Source: CAD feature listing. Evaluate the final solid. Frame: model axes, mm. Face numbers are marked on the shaded views. A direction names the side the tool comes from. Give positions to 0.01 mm unless a question says otherwise; leave off trailing zeros. Order: outer loops, then holes, each group sorted by start corner. A loop starts at its lowest first (then second) coordinate and runs counter-clockwise, first axis right, second up. Notation, with made-up numbers: M -22.5,33 L 34.5,33 A37 cw 34.5,69 Z; hole C 14.5,-28.5 d1. An arc over 180 degrees is marked long. Return JSON: item names as keys, results as strings.
from build123d import *
from build123d.topology import SkipClean

# Parameters (mm, degrees)
BOSS_EXTRUDE1_DEPTH = 19
SKETCH2_R           = 2.1
BOSS_EXTRUDE2_DEPTH = 1
SKETCH3_R           = 4.5
BOSS_EXTRUDE3_DEPTH = 1.5
SKETCH4_R           = 2.5
BOSS_EXTRUDE4_DEPTH = 2.5
BOSS_EXTRUDE5_DEPTH = 6


with BuildPart() as part:
    # Sketch1 → Boss-Extrude1 (new body)
    with BuildSketch(Plane(origin=(0, 0, 0), x_dir=(1, 0, 0), z_dir=(0, 1, 0))):
        with BuildLine():
            Line((-7.4, -17), (-7.4, -11.884443613))
            ThreePointArc((-7.4, -11.884443613), (0, 14), (7.4, -11.884443613))
            Line((7.4, -11.884443613), (7.4, -17))
            Line((7.4, -17), (-7.4, -17))
        make_face()
    extrude(amount=BOSS_EXTRUDE1_DEPTH)

    # Sketch2 → Boss-Extrude2 (add)
    # profile 1 of 2: a face of its own
    with BuildSketch(Plane.XZ):
        with BuildLine():
            Line((13.555441712, -3.5), (13.555441712, 3.5))
            Line((13.555441712, 3.5), (17.5, 3.5))
            ThreePointArc((17.5, 3.5), (21, 0), (17.5, -3.5))
            Line((17.5, -3.5), (13.555441712, -3.5))
        make_face()
        with Locations(Location((17.5, 0, 0), (0, 0, 90))):
            Circle(SKETCH2_R, mode=Mode.SUBTRACT)
    # profile 2 of 2: a face of its own
    with BuildSketch(Plane.XZ):
        with BuildLine():
            Line((-17.5, -3.5), (-13.555441712, -3.5))
            Line((-13.555441712, -3.5), (-13.555441712, 3.5))
            Line((-13.555441712, 3.5), (-17.5, 3.5))
            ThreePointArc((-17.5, 3.5), (-21, 0), (-17.5, -3.5))
        make_face()
        with Locations(Location((-17.5, 0, 0), (0, 0, 270))):
            Circle(SKETCH2_R, mode=Mode.SUBTRACT)
    extrude(amount=-BOSS_EXTRUDE2_DEPTH)

    # Sketch3 → Boss-Extrude3 (add)
    with BuildSketch(Plane.XZ):
        with Locations(Location((0, -8, 0), (0, 0, 90))):
            Circle(SKETCH3_R)
    extrude(amount=BOSS_EXTRUDE3_DEPTH)

    # Sketch4 → Boss-Extrude4 (add)
    with BuildSketch(Plane.XZ.offset(1.5)):
        with Locations(Location((0, -8, 0), (0, 0, 270))):
            Circle(SKETCH4_R)
    extrude(amount=BOSS_EXTRUDE4_DEPTH)

    # Sketch5 → Boss-Extrude5 (add)
    with SkipClean():  # the faces are left unmerged after this step: merging them gives an invalid solid
        with BuildSketch(Plane.XZ.offset(4)):
            with BuildLine():
                Line((-1.5, -10), (-1.5, -6))
                ThreePointArc((-1.5, -6), (0, -5.5), (1.5, -6))
                Line((1.5, -6), (1.5, -10))
                ThreePointArc((1.5, -10), (0, -10.5), (-1.5, -10))
            make_face()
        extrude(amount=BOSS_EXTRUDE5_DEPTH)


solid = part.part
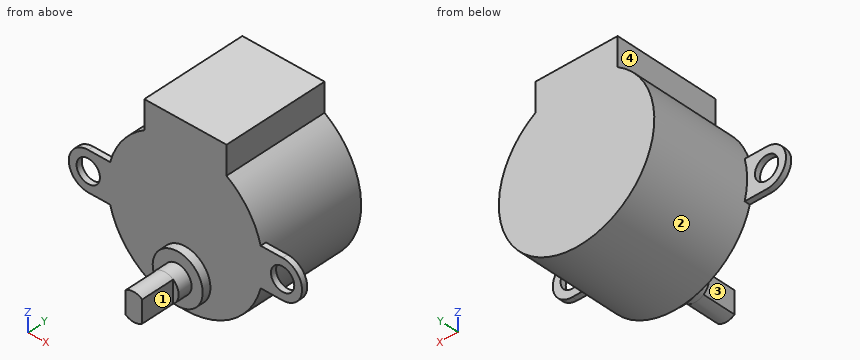
1. First-contact query: pin 1 (8 mm diameter, centred on y = 14.5, z = 4, fed in from -X); pin 2 (2 mm diameter, centred on y = -6, z = -8, fed in from +X); pin 3 (1.2 mm diameter, centred on y = -8.5, z = -8, fed in from -X). Flat tips, straight axial feed; report the tip coordinate or a pass-through.
Evaluation:
{"pin 1": "stops at x = -14", "pin 2": "stops at x = 1.5", "pin 3": "stops at x = -1.5"}
2. Section query C-C (x = -4). Return loops of the section in (y, z).
Evaluation:
{"outline": "M -1.5,-10.06 L 0,-10.06 L 0,-13.42 L 19,-13.42 L 19,17 L 0,17 L 0,-5.94 L -1.5,-5.94 Z"}
3. Ray query, probe 1 along X at (y, z) = (0.5, 0); probe 2 along Z at (x, y) = (17.5, 0.3); probe 3 along Y at (x, z) = (-2, -1). Return the intervals inside material, ascending.
Evaluation:
{"probe 1": "x = -21 to -19.6, -15.4 to 15.4, 19.6 to 21", "probe 2": "z = -3.5 to -2.1, 2.1 to 3.5", "probe 3": "y = 0 to 19"}
4. Section query B-B (y = 12.25). Return loops of the section in (x, z), then the cut area to 3 significant figures.
Evaluation:
{"outline": "M -7.4,11.88 A14 ccw long 7.4,11.88 L 7.4,17 L -7.4,17 Z", "area": "670 mm^2"}
5. Section query D-D (z = -8). Return loops of the section in (x, y), then the cut area to 3 significant figures.
Evaluation:
{"outline": "M -11.49,0 L -4.5,0 L -4.5,-1.5 L -2.5,-1.5 L -2.5,-4 L -1.5,-4 L -1.5,-10 L 1.5,-10 L 1.5,-4 L 2.5,-4 L 2.5,-1.5 L 4.5,-1.5 L 4.5,0 L 11.49,0 L 11.49,19 L -11.49,19 Z", "area": "481 mm^2"}
6. Section query A-A (z = 0). Return loops of the section in (x, y).
Evaluation:
{"outline": "M -21,0 L -19.6,0 L -19.6,1 L -21,1 Z; M -15.4,0 L 15.4,0 L 15.4,1 L 14,1 L 14,19 L -14,19 L -14,1 L -15.4,1 Z; M 19.6,0 L 21,0 L 21,1 L 19.6,1 Z"}
7. Set-up query: the marked faces 1, 2, 3 and 4. Return all of +Z, -Z, +X, -X, +Y, -Y with unobstructed straight access to the full face (end or side cutting, diameter ignored); none if empty.
Evaluation:
{"face 1": "+Z, -Z, +X, -Y", "face 2": "+Y", "face 3": "+Z, -Z, -X, -Y", "face 4": "+Z, -X, +Y, -Y"}
